Input: part model. Units: mm. Frame: model coordinates. Face numbers are marked on the shaded views. A direction names the side the tool comes from. Round coordinates to 2 decimals unless told otherwise and drop trailing zeros. Write each loop counter-clockwise with the first axis right and the second up, starting at its lowest first coordinate (ties: lowest second). Pieces come first, ordered by that corner, then holes. Notation, with made-up numbers: (-18, 17) -> (-11, 17) arc R12 cw to (-11, 28) -> close; hole circle Ø1 at (-12.75, -13.75). An arc over 180 degrees is marked (long way). Use CSV: the item, a comma, the result in double quotes.
```python
from build123d import *

# Parameters (mm, degrees)
F1_DEPTH = 2
F2_W     = 48.26
F2_H     = 2
F3_DEPTH = 33.56
F5_D     = 3.81
F6_R     = 5.08
F7_D     = 2


with BuildPart() as f1:
    # F0 (on Top) → F1 (new body)
    with BuildSketch(Plane.XY):
        with BuildLine():
            ThreePointArc((0, -11.94943), (8.449523, -8.449523), (11.94943, 0))
            ThreePointArc((11.94943, 0), (0, 11.94943), (-11.94943, 0))
            ThreePointArc((-11.94943, 0), (-8.449523, -8.449523), (0, -11.94943))
        make_face()
        with BuildLine():
            ThreePointArc((0, 3.5), (2.474874, 2.474874), (3.5, 0))
            ThreePointArc((3.5, 0), (2.474874, -2.474874), (0, -3.5))
            ThreePointArc((0, -3.5), (-2.474874, -2.474874), (-3.5, 0))
            ThreePointArc((-3.5, 0), (-2.474874, 2.474874), (0, 3.5))
        make_face(mode=Mode.SUBTRACT)
        with BuildLine():
            Line((11.94943, -11.94943), (11.94943, 0))
            ThreePointArc((11.94943, 0), (8.449523, -8.449523), (0, -11.94943))
            Line((0, -11.94943), (11.94943, -11.94943))
        make_face()
        with BuildLine():
            ThreePointArc((0, -11.94943), (-8.449523, -8.449523), (-11.94943, 0))
            Line((-11.94943, 0), (-11.94943, -11.94943))
            Line((-11.94943, -11.94943), (0, -11.94943))
        make_face()
        Polygon((11.94943, -11.94943), (0, -11.94943), (-11.94943, -11.94943), (-24.13, -11.94943), (-24.13, -13.94943), (24.13, -13.94943), (24.13, -11.94943), align=None)
    extrude(amount=-F1_DEPTH)

    # F2 (on face) → F3 (join)
    with BuildSketch(Plane.XY):
        with Locations((0, -12.94943)):
            Rectangle(F2_W, F2_H)
    extrude(amount=F3_DEPTH)

    # F5 (through all)
    with Locations(Plane.XZ.offset(13.94943)):
        with Locations((-14.224, 29.496), (14.224, 29.496), (14.224, 2.064), (-14.224, 2.064)):
            Hole(F5_D / 2)

    # F6
    f6_edges = [f1.edges().sort_by_distance(p)[0] for p in [
        (24.13, -12.94943, 33.56),
        (-24.13, -12.94943, 33.56),
        (-24.13, -12.94943, -2),
        (24.13, -12.94943, -2),
    ]]
    fillet(f6_edges, radius=F6_R)

    # F7 (through all)
    with Locations(Plane.XY):
        with Locations((0, -8.5), (8.5, 0), (-8.5, 0), (0, 8.5)):
            Hole(F7_D / 2)


solid = f1.part
```
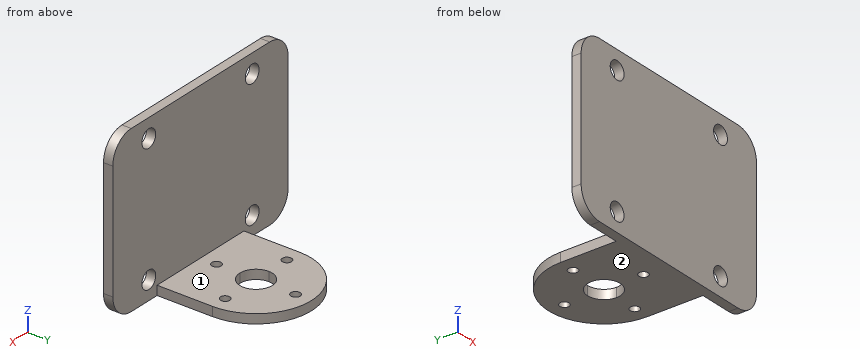
Item 1: Section query D-D on y = 8.5. Return the cut outline in (x, z).
Worked answers:
outline,"(-8.4, -2) -> (-1, -2) -> (-1, 0) -> (-8.4, 0) -> close; (1, -2) -> (8.4, -2) -> (8.4, 0) -> (1, 0) -> close"
Item 2: Section query B-B on x = -8.5. Return the cut outline in (y, z), plus the area to 3 significant figures.
Worked answers:
outline,"(-13.95, -2) -> (-1, -2) -> (-1, 0) -> (-11.95, 0) -> (-11.95, 33.56) -> (-13.95, 33.56) -> close; (1, -2) -> (8.4, -2) -> (8.4, 0) -> (1, 0) -> close"
area,"108 mm²"
Item 3: First-contact query: pin 1 Ø2.5 at (x, y) = (8.5, 0) entering from +Z; pin 2 Ø4 at (x, z) = (-1.5, 10) entering from +Y; pin 3 Ø1 at (y, z) = (-3.5, -1.5) entering from +X. Flat tips, straight axial feed; report the tip coordinate or a pass-through.
Worked answers:
pin 1,"stops at z = 0"
pin 2,"stops at y = -11.95"
pin 3,"stops at x = 11.95"
Item 4: Set-up query: the marked faces 1 and 2. Return all of +Z, -Z, +X, -X, +Y, -Y with unobstructed straight access to the full face (end or side cutting, diameter ignored); none if empty.
Worked answers:
face 1,"+Z, +X, -X, +Y"
face 2,"-Z, +X, -X, +Y, -Y"
Item 5: Line query: line 1 (X direction, y = -12.5, z = 30); line 2 (Y direction, x = -11.5, z = 16); line 3 (Z direction, x = 9, y = 1). Output: solid intervals per line, ascending.
Worked answers:
line 1,"x = -23.9 to -16.06, -12.39 to 12.39, 16.06 to 23.9"
line 2,"y = -13.95 to -11.95"
line 3,"z = -2 to 0"
Item 6: Section query C-C on z = 10. Return the cut outline in (x, y), plus the area to 3 significant figures.
Worked answers:
outline,"(-24.13, -13.95) -> (24.13, -13.95) -> (24.13, -11.95) -> (-24.13, -11.95) -> close"
area,"96.5 mm²"
Item 7: Section query A-A on y = -8.5. Return the cut outline in (x, z).
Worked answers:
outline,"(-11.95, -2) -> (-1, -2) -> (-1, 0) -> (-11.95, 0) -> close; (1, -2) -> (11.95, -2) -> (11.95, 0) -> (1, 0) -> close"
